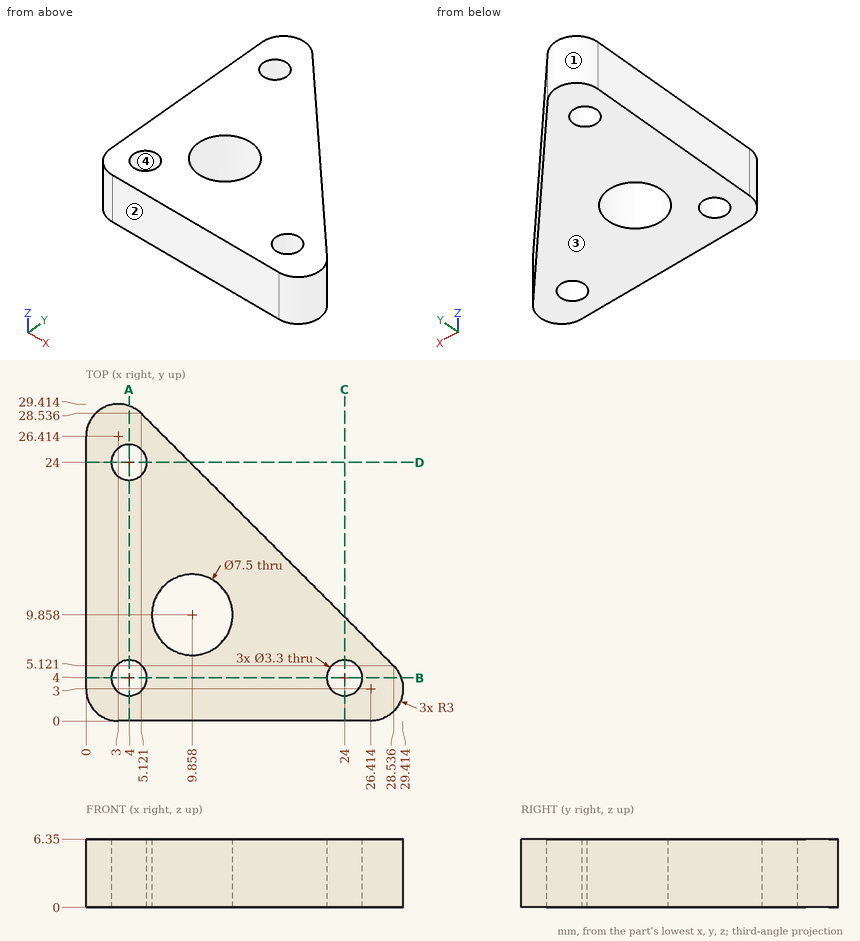
The drawing under review shows one solid part. Ordinate dimensions are in mm from its lowest x, y, z. Round coordinates to 2 decimals unless told otherwise and drop trailing zeros. Loops run counter-clockwise (first coordinate to the right, second up) from the corner with the lowest first, then second, coordinate; pieces in that order, holes last. Notation, with made-up numbers: (-17, 62) - (13, 62) arc R17 ccw to (13, 92) - close; hole circle Ø1 at (-15.75, 58.25). An arc over 180 degrees is marked (long way). Put each result on its own line as item: value. Start each with the question number.
1. Consider section C-C on x = 24. State the section outline as (y, z) points.
2. Consider section A-A on x = 4. State the section outline as (y, z) points, plus the area to 3 significant figures.
3. Mouldability with a two-part tool opening along Y and no side actions: class the marked faces 1, 2, 3 and 4 as +Y half, -Y half, draft (parallel to the pull), parting line (faces both ways), or undercut.
4. Insertion check: P1, Ø1.5, axis at y = 5.5, z = 5, coming from the +X side. The pin has a flat end and moves straight along its axis. Give the tip position at first contact, or say it passes through.
5. For probe 1 along Y at (x, z) = (4.5, 2.25); probe 2 along Y at (x, z) = (4, 1.25); probe 3 along X at (y, z) = (3.5, 3.25), list the stretches that pass through material, from the lowest coordinate up. Write a range as [from, to].
Result sheet:
1. outline: (0, 0) - (2.35, 0) - (2.35, 6.35) - (0, 6.35) - close; (5.65, 0) - (9.66, 0) - (9.66, 6.35) - (5.65, 6.35) - close
2. outline: (0, 0) - (2.35, 0) - (2.35, 6.35) - (0, 6.35) - close; (5.65, 0) - (22.35, 0) - (22.35, 6.35) - (5.65, 6.35) - close; (25.65, 0) - (29.24, 0) - (29.24, 6.35) - (25.65, 6.35) - close
2. area: 144 mm^2
3. face 1: +Y half
3. face 2: -Y half
3. face 3: draft
3. face 4: undercut
4. P1: x = 28.85
5. probe 1: [0, 2.43], [5.57, 22.43], [25.57, 29.01]
5. probe 2: [0, 2.35], [5.65, 22.35], [25.65, 29.24]
5. probe 3: [0, 2.43], [5.57, 22.43], [25.57, 29.37]
